Verification items for the finished model (mm, model axes). A direction names the side the tool comes from. Round coordinates to 2 decimals unless told otherwise and drop trailing zeros. Write each loop counter-clockwise with the first axis right and the second up, starting at its lowest first coordinate (ties: lowest second). Pieces come first, ordered by that corner, then holes.
from build123d import *

# Parameters (mm, degrees)
ESQUISSE1_R              = 15
ESQUISSE1_R_2            = 5
BOSS_EXTRU_4_DEPTH       = 10
ESQUISSE3_R              = 50
BOSS_EXTRU_5_DEPTH       = 10
ESQUISSE14_R             = 5
ENL_V_MAT_EXTRU_1_DEPTH  = 10
ENL_V_MAT_EXTRU_7_DEPTH  = 10
ENL_V_MAT_EXTRU_8_REACH  = 52
ESQUISSE20_R             = 2.25
ESQUISSE25_W             = 7
ESQUISSE25_H             = 3.5
ENL_V_MAT_EXTRU_10_DEPTH = 10


with BuildPart() as part:
    # Esquisse1 → Boss.-Extru.4 (new body)
    with BuildSketch(Plane.XY):
        Circle(ESQUISSE1_R)
        Circle(ESQUISSE1_R_2, mode=Mode.SUBTRACT)
    extrude(amount=BOSS_EXTRU_4_DEPTH)

    # Esquisse3 → Boss.-Extru.5 (add)
    with BuildSketch(Plane.XY):
        Circle(ESQUISSE3_R)
    extrude(amount=-BOSS_EXTRU_5_DEPTH)

    # Esquisse14 → Enlèv. mat.-Extru.1 (cut)
    with BuildSketch(Plane.XY):
        Circle(ESQUISSE14_R)
    extrude(amount=-ENL_V_MAT_EXTRU_1_DEPTH, mode=Mode.SUBTRACT)

    # Esquisse19 → Enlèv. mat.-Extru.7 (cut)
    with BuildSketch(Plane.XY):
        with BuildLine():
            Line((-13.338573188, -9.521928054), (-27.218975217, -26.077663465))
            ThreePointArc((-27.218975217, -26.077663465), (-30.359478039, -27.507055347), (-33.443966468, -25.96049456))
            ThreePointArc((-33.443966468, -25.96049456), (-40.74820108, -11.49044297), (-42.079621744, 4.663861575))
            ThreePointArc((-42.079621744, 4.663861575), (-40.257507229, 7.594018196), (-36.832899826, 8.015898828))
            Line((-36.832899826, 8.015898828), (-16.348106085, 1.150685003))
            ThreePointArc((-16.348106085, 1.150685003), (-15.386221176, 0.457781948), (-14.985564031, -0.65792907))
            ThreePointArc((-14.985564031, -0.65792907), (-14.436989432, -4.07103625), (-13.121635222, -7.267921925))
            ThreePointArc((-13.121635222, -7.267921925), (-12.88038592, -8.428583804), (-13.338573188, -9.521928054))
        make_face()
        with BuildLine():
            Line((-13.177737519, 9.74329936), (-33.212457679, 17.828342562))
            ThreePointArc((-33.212457679, 17.828342562), (-35.542358886, 20.373431853), (-35.024651516, 23.784868238))
            ThreePointArc((-35.024651516, 23.784868238), (-23.519947285, 35.203100014), (-8.567722294, 41.461310949))
            ThreePointArc((-8.567722294, 41.461310949), (-5.217913395, 40.633845258), (-3.758419184, 37.507218357))
            Line((-3.758419184, 37.507218357), (-3.957476136, 15.903554042))
            ThreePointArc((-3.957476136, 15.903554042), (-4.319227318, 14.774628312), (-5.256521685, 14.048807059))
            ThreePointArc((-5.256521685, 14.048807059), (-8.333060636, 12.472373489), (-10.967012784, 10.233505294))
            ThreePointArc((-10.967012784, 10.233505294), (-11.996317693, 9.645399328), (-13.177737519, 9.74329936))
        make_face()
        with BuildLine():
            Line((5.194283506, 15.543618221), (6.692547521, 37.096185131))
            ThreePointArc((6.692547521, 37.096185131), (8.393092207, 40.098528699), (11.797541387, 40.660351549))
            ThreePointArc((11.797541387, 40.660351549), (26.212074244, 33.247155288), (36.78447816, 20.96063781))
            ThreePointArc((36.78447816, 20.96063781), (37.032659401, 17.519079267), (34.510069026, 15.16483694))
            Line((34.510069026, 15.16483694), (13.902251323, 8.678251937))
            ThreePointArc((13.902251323, 8.678251937), (12.716791888, 8.67344052), (11.736854967, 9.340569333))
            ThreePointArc((11.736854967, 9.340569333), (9.286874729, 11.779386986), (6.343648566, 13.59257602))
            ThreePointArc((6.343648566, 13.59257602), (5.466253846, 14.389768423), (5.194283506, 15.543618221))
        make_face()
        with BuildLine():
            Line((-19.005564812, -32.553120431), (-6.146209076, -15.1923916))
            ThreePointArc((-6.146209076, -15.1923916), (-5.189980327, -14.491703509), (-4.005066227, -14.455429586))
            ThreePointArc((-4.005066227, -14.455429586), (-0.589489528, -14.988412261), (2.857396229, -14.725328071))
            ThreePointArc((2.857396229, -14.725328071), (4.035801406, -14.854550596), (4.934045928, -15.628174536))
            Line((4.934045928, -15.628174536), (16.390205856, -33.945224931))
            ThreePointArc((16.390205856, -33.945224931), (16.779169577, -37.373726988), (14.35514352, -39.829336241))
            ThreePointArc((14.35514352, -39.829336241), (-1.663825962, -42.304584315), (-17.438914178, -38.578885977))
            ThreePointArc((-17.438914178, -38.578885977), (-19.662594375, -35.940483902), (-19.005564812, -32.553120431))
        make_face()
        with BuildLine():
            Line((16.387981273, -0.136814991), (37.348679518, 5.098360702))
            ThreePointArc((37.348679518, 5.098360702), (40.729575141, 4.408821782), (42.315933076, 1.344611014))
            ThreePointArc((42.315933076, 1.344611014), (39.719900084, -14.655228017), (31.301780055, -28.506924356))
            ThreePointArc((31.301780055, -28.506924356), (28.105355598, -29.80645882), (25.086814797, -28.134833694))
            Line((25.086814797, -28.134833694), (12.549539974, -10.540099382))
            ThreePointArc((12.549539974, -10.540099382), (12.178636933, -9.414147271), (12.510296976, -8.276017736))
            ThreePointArc((12.510296976, -8.276017736), (14.072664867, -5.192311964), (14.887603211, -1.832831318))
            ThreePointArc((14.887603211, -1.832831318), (15.374648361, -0.752033352), (16.387981273, -0.136814991))
        make_face()
    extrude(amount=-ENL_V_MAT_EXTRU_7_DEPTH, mode=Mode.SUBTRACT)

    # Esquisse20 → Enlèv. mat.-Extru.8 (cut, up to next)
    with BuildSketch(Plane(origin=(0, 0, 0), x_dir=(1, 0, 0), z_dir=(0, 1, 0)), mode=Mode.PRIVATE) as enl_v_mat_extru_8_sk1:
        with Locations((0, -5)):
            Circle(ESQUISSE20_R)
    enl_v_mat_extru_8_tool1 = extrude(enl_v_mat_extru_8_sk1.sketch, amount=ENL_V_MAT_EXTRU_8_REACH, mode=Mode.PRIVATE) & part.part
    add(enl_v_mat_extru_8_tool1.solids().sort_by_distance((0, 0, 5))[0], mode=Mode.SUBTRACT)

    # Esquisse25 → Enlèv. mat.-Extru.10 (cut)
    with BuildSketch(Plane.XY):
        with Locations((0, 10)):
            Rectangle(ESQUISSE25_W, ESQUISSE25_H)
    extrude(amount=ENL_V_MAT_EXTRU_10_DEPTH, mode=Mode.SUBTRACT)


solid = part.part
Q1. Material ranges on line 1 along Y through (x, z) = (0, 1); line 2 along X through (y, z) = (-21, -6); line 3 along Z through (x, y) = (0, 6.35), recorded low to high.
Recorded:
line 1: y = -15 to -5, 5 to 8.25, 11.75 to 15
line 2: x = -45.38 to -36.76, -22.96 to -10.45, 8.29 to 20, 36.76 to 45.38
line 3: z = -10 to 2.75, 7.25 to 10
Q2. Sectioned sample at D-D (z = -1.25). Give the number of separate pieces and of enclosed holes in the cut face, plus the area to 3 significant figures.
Recorded:
separate pieces: 1
enclosed holes: 6
area: 4,270 mm2
Q3. Sectioned sample at A-A (x = 0). Enter the section's corners in (y, z), plus the area to 3 significant figures.
Recorded:
outline: (-50, -10) - (-42.34, -10) - (-42.34, 0) - (-50, 0) - close; (-15, -10) - (-5, -10) - (-5, 10) - (-15, 10) - close; (5, -10) - (50, -10) - (50, 0) - (15, 0) - (15, 2.75) - (11.75, 2.75) - (11.75, 0) - (8.25, 0) - (8.25, 2.75) - (5, 2.75) - close; (5, 7.25) - (8.25, 7.25) - (8.25, 10) - (5, 10) - close; (11.75, 7.25) - (15, 7.25) - (15, 10) - (11.75, 10) - close
area: 762 mm2
Q4. Tool access check on faces 4 (the flat face through (-0.8, 8.25, 2.7)), 5 (the flat face through (-23.055, 13.729, -4.93)). Record the directions out of +Z, -Z, +X, -X, +Y, -Y that give a thin tool (end or side, any length) a straight path to the whole face; none if there is none.
Recorded:
face 4: +Z
face 5: +Z, -Z
Q5. Sectioned sample at B-B (x = 32.5). Enter the section's corners in (y, z), plus the area to 3 significant figures.
Recorded:
outline: (-38, -10) - (-27.13, -10) - (-27.13, 0) - (-38, 0) - close; (3.89, -10) - (14.53, -10) - (14.53, 0) - (3.89, 0) - close; (27.13, -10) - (38, -10) - (38, 0) - (27.13, 0) - close
area: 324 mm2
Q6. Release check for a two-part mould opening along Y. For faces 1 (the flat face through (-4, 4, 10)), 2 (the cylindrical face through (8.35, 40.07, -4.93)), 3 (the flat face through (-20.18, -17.68, -4.93)) record: released by +Y, released by -Y, zero draft, split by the parting line, or undercut.
Recorded:
face 1: zero draft
face 2: undercut
face 3: undercut
Q7. Sectioned sample at C-C (z = 5). Enter the section's corners in (x, y), plus the area to 3 significant figures.
Recorded:
outline: (-3.5, 8.25) - (-3.5, 11.75) - (-2.25, 11.75) - (-2.25, 14.83) arc R15 ccw (long way) to (2.25, 14.83) - (2.25, 11.75) - (3.5, 11.75) - (3.5, 8.25) - (2.25, 8.25) - (2.25, 4.47) arc R5 cw (long way) to (-2.25, 4.47) - (-2.25, 8.25) - close
area: 574 mm2
Q8. Depth check by flat-ended pin: P1, Ø7.5, axis at x = -1, z = 4.5, coming from the +Y side; P2, Ø8, axis at x = -4, z = -2, coming from the +Y side; P3, Ø5, axis at x = 14, z = -7, coming from the -Y side; P4, Ø13, axis at x = 0, y = 0, coming from the +Z side. Enter the tip coordinate at first touch or a pass-through.
Recorded:
P1: stops at y = 15
P2: stops at y = 50
P3: stops at y = -48.66
P4: stops at z = 10
